Could you check a few things on this drawing? It's one solid part, dimensions in mm from its lowest x, y, z. A direction names the side the tool comes from. Give positions to 0.01 mm unless a question says otherwise; leave off trailing zeros. Order: outer loops, then holes, each group sorted by start corner. A loop starts at its lowest first (then second) coordinate and runs counter-clockwise, first axis right, second up.
(1) Will these pins go through, and if not, where does the flat tip stop? pin 1 (3 mm diameter, centred on x = 24.5, z = 4, fed in from -Y); pin 2 (2.5 mm diameter, centred on y = 2, z = 3.5, fed in from +X); pin 3 (0.6 mm diameter, centred on x = 116.5, z = 2, fed in from +Y).
(2) Imagine slicing it at B-B, the plane x = 110.5. Write out the boundary of the cut face in (y, z).
(3) If I drill on probe 1 along X at (y, z) = (10.5, 1.4); probe 2 along X at (y, z) = (5, 4.8); probe 3 along Y at (x, z) = (47, 0.35), over which ranges is the centre line in solid material (lowest first)?
(4) Imagine slicing it at A-A, the plane z = 3.5. Write out the boundary of the cut face in (x, y).
(5) On a 3-axis mill with a long thin cutter (end or side, diameter ignored), from which of +Z, -Z, +X, -X, +Y, -Y can I reach the whole of each face in a straight line? I mean the marked faces 1 and 2. Say none if no direction works.
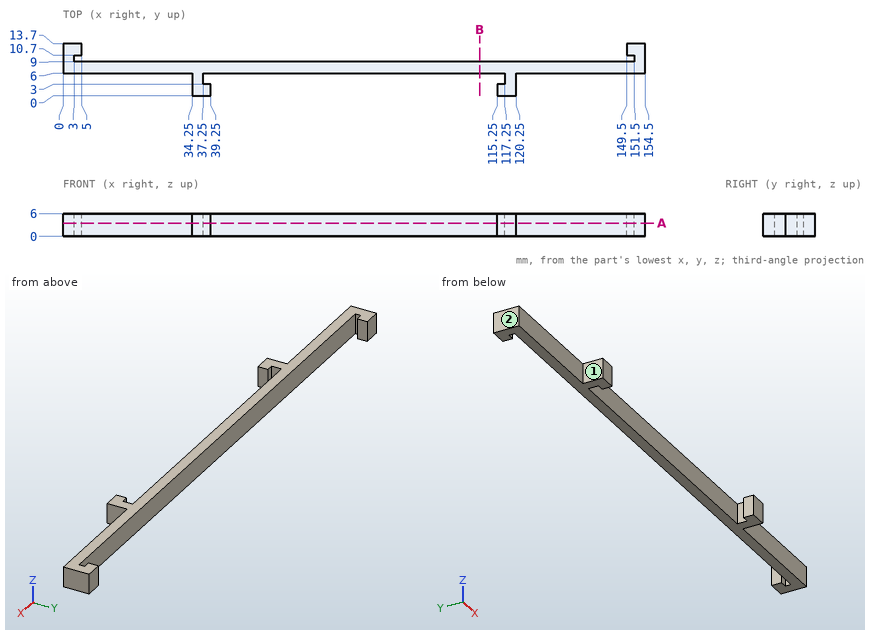
Answer block:
1. pin 1: stops at y = 6
1. pin 2: stops at x = 120.25
1. pin 3: stops at y = 9
2. outline: (6, 0) - (9, 0) - (9, 6) - (6, 6) - close
3. probe 1: x = 0 to 3, 151.5 to 154.5
3. probe 2: x = 34.25 to 37.25, 117.25 to 120.25
3. probe 3: y = 6 to 9
4. outline: (0, 6) - (34.25, 6) - (34.25, 0) - (39.25, 0) - (39.25, 3) - (37.25, 3) - (37.25, 6) - (117.25, 6) - (117.25, 3) - (115.25, 3) - (115.25, 0) - (120.25, 0) - (120.25, 6) - (154.5, 6) - (154.5, 13.7) - (149.5, 13.7) - (149.5, 10.7) - (151.5, 10.7) - (151.5, 9) - (3, 9) - (3, 10.7) - (5, 10.7) - (5, 13.7) - (0, 13.7) - close
5. face 1: +Z, -Z, -X, -Y
5. face 2: +Z, -Z, -X, +Y, -Y
